from build123d import *

# Parameters (mm, degrees)
SKETCH1_W           = 3.05
SKETCH1_H           = 2.41
BOSS_EXTRUDE1_DEPTH = 8.5
CUT_EXTRUDE1_START  = 8.5
SKETCH1_3_W         = 0.64
SKETCH1_3_H         = 0.64
CUT_EXTRUDE1_DEPTH  = 5
CHAMFER1_SIZE       = 0.5
SKETCH2_W           = 3.2
SKETCH2_H           = 0.64
BOSS_EXTRUDE2_DEPTH = 0.32
CHAMFER2_SIZE       = 0.2


with BuildPart() as part:
    # Sketch1 → Boss-Extrude1 (new body)
    with BuildSketch(Plane.XY):
        Rectangle(SKETCH1_W, SKETCH1_H)
    extrude(amount=BOSS_EXTRUDE1_DEPTH)

    # Sketch1<3> → Cut-Extrude1 (cut)
    with BuildSketch(Plane.XY.offset(CUT_EXTRUDE1_START)):
        Rectangle(SKETCH1_3_W, SKETCH1_3_H)
    extrude(amount=-CUT_EXTRUDE1_DEPTH, mode=Mode.SUBTRACT)

    # Chamfer1
    chamfer1_edges = [part.edges().sort_by_distance(p)[0] for p in [
        (-0.32, 0, 8.5),
        (0, -0.32, 8.5),
        (0.32, 0, 8.5),
        (0, 0.32, 8.5),
    ]]
    chamfer(chamfer1_edges, length=CHAMFER1_SIZE)

    # Sketch2 → Boss-Extrude2 (add, symmetric)
    with BuildSketch(Plane(origin=(0, 0, 0), x_dir=(0, 0, -1), z_dir=(1, 0, 0))):
        with Locations((1.6, 0)):
            Rectangle(SKETCH2_W, SKETCH2_H)
    extrude(amount=BOSS_EXTRUDE2_DEPTH, both=True)

    # Chamfer2
    chamfer2_edges = [part.edges().sort_by_distance(p)[0] for p in [
        (0.32, 0, -3.2),
        (0, -0.32, -3.2),
        (0, 0.32, -3.2),
        (-0.32, 0, -3.2),
    ]]
    chamfer(chamfer2_edges, length=CHAMFER2_SIZE)


solid = part.part
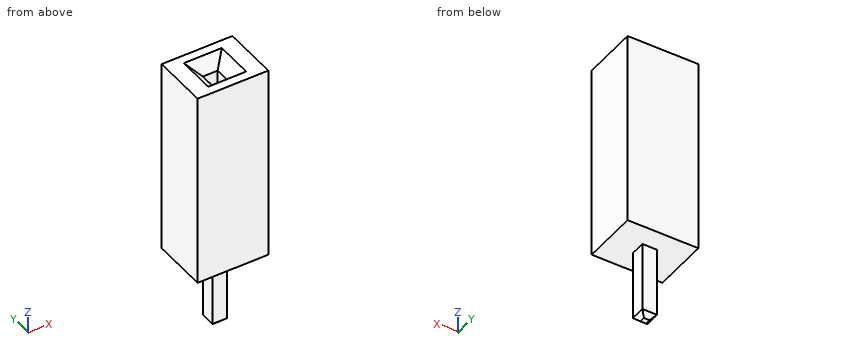
Geometry: final body of the model. Coordinates: model frame, mm. Give positions to 0.01 mm unless a question says otherwise; leave off trailing zeros. Order: outer loops, then holes, each group sorted by start corner. A loop starts at its lowest first (then second) coordinate and runs counter-clockwise, first axis right, second up. Notation, with made-up numbers: (11.25, -31.5) -> (17.25, -31.5) arc R23 cw to (17.25, -7.5) -> close; hole circle Ø9 at (88, 51). An arc over 180 degrees is marked (long way). Put each result on its own line as item: value.
Q1. Material intervals for L1, parallel to Y at x = 0.2, z = 7 (3 decimals); L2, parallel to X at y = 0.1, z = 7.25 (3 decimals); L3, parallel to Z at x = 0.9, y = -0.8, sorted ascending.
Here are the results:
L1: y = -1.205 to -0.32, 0.32 to 1.205
L2: x = -1.525 to -0.32, 0.32 to 1.525
L3: z = 0 to 8.5
Q2. Section B-B, the plane y = -0.45. Return loops of the section in (x, z) (3 decimals).
Here are the results:
outline: (-1.525, 0) -> (1.525, 0) -> (1.525, 8.5) -> (0.82, 8.5) -> (0.45, 8.13) -> (-0.45, 8.13) -> (-0.82, 8.5) -> (-1.525, 8.5) -> close
Q3. Pin query (flat end, axial travel): pin 1 (0.7 mm diameter, centred on x = -0.5, y = 0, fed in from -Z); pin 2 (0.5 mm diameter, centred on y = 0, z = -1, fed in from -X); pin 3 (0.7 mm diameter, centred on x = 0, z = -1.5, fed in from -Y). Return the tip coordinate at first contact, or that it passes through.
Here are the results:
pin 1: stops at z = -3.17
pin 2: stops at x = -0.32
pin 3: stops at y = -0.32
Q4. Section A-A, the plane z = 7.75. Return loops of the section in (x, y) (3 decimals), then the cut area to 3 significant figures.
Here are the results:
outline: (-1.525, -1.205) -> (1.525, -1.205) -> (1.525, 1.205) -> (-1.525, 1.205) -> close; hole (-0.32, -0.32) -> (0.32, -0.32) -> (0.32, 0.32) -> (-0.32, 0.32) -> close
area: 6.94 mm^2
Q5. Section D-D, the plane z = -0.25. Return loops of the section in (x, y), then the cut area to 3 significant figures.
Here are the results:
outline: (-0.32, -0.32) -> (0.32, -0.32) -> (0.32, 0.32) -> (-0.32, 0.32) -> close
area: 0.410 mm^2
Q6. Section C-C, the plane x = 0.55. Return loops of the section in (y, z) (3 decimals).
Here are the results:
outline: (-1.205, 0) -> (1.205, 0) -> (1.205, 8.5) -> (0.82, 8.5) -> (0.55, 8.23) -> (-0.55, 8.23) -> (-0.82, 8.5) -> (-1.205, 8.5) -> close
